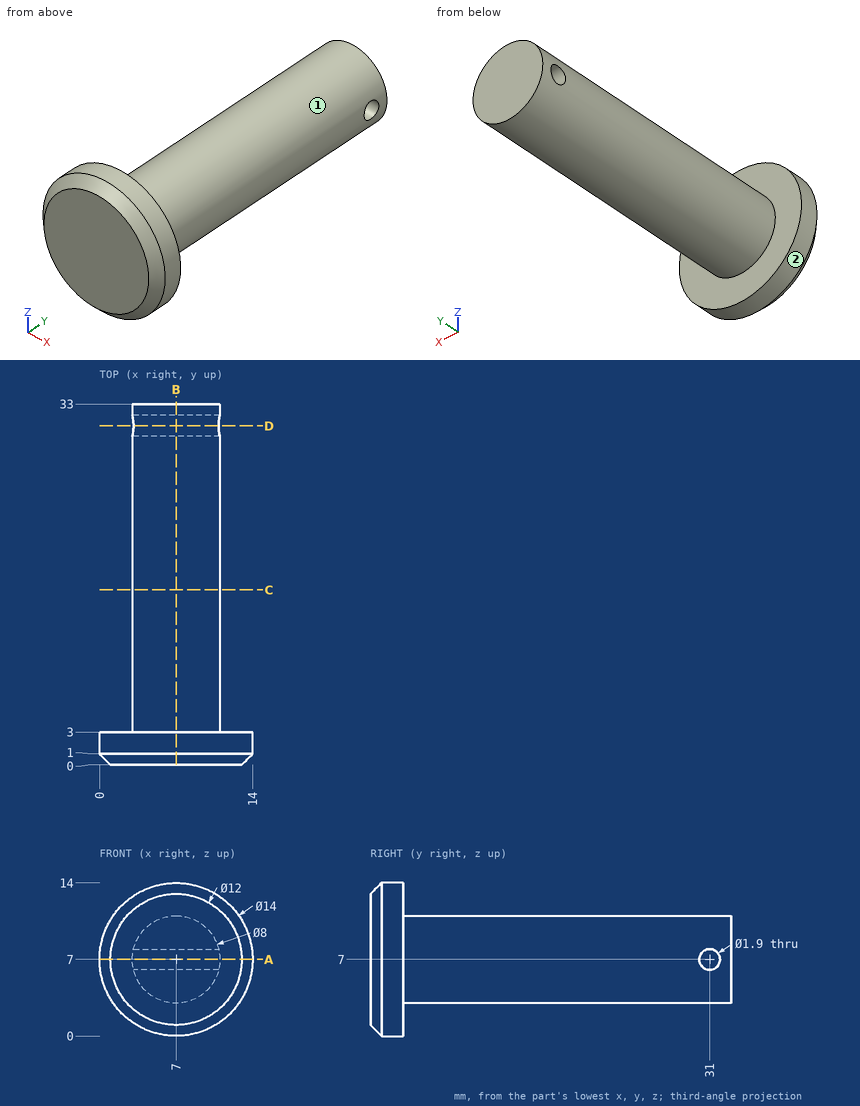
Study the drawing (mm; zero at the part's minimum x, y, z) and answer. A direction names the side the tool comes from. Coordinates: 2 decimals unless noted, no trailing zeros. Loops run counter-clockwise (first coordinate to the right, second up) from the corner with the lowest first, then second, coordinate; pieces in that order, holes last. Notation, with made-up numbers: (14, 21.25) -> (25, 21.25) arc R29 ccw to (25, 56.25) -> close; hole circle Ø9 at (27, 69). An arc over 180 degrees is marked (long way). Answer in a Markdown table with one row per item. Add a question column.
1. The part is cut by section A-A, the plane z = 7. Write down the section's boundary in (x, y).
2. The part is cut by section C-C, the plane y = 16. Write down the section's boundary in (x, z), then the cut area to 3 significant figures.
3. The part is cut by section B-B, the plane x = 7. Write down the section's boundary in (y, z).
4. The part is cut by section D-D, the plane y = 31. Write down the section's boundary in (x, z).
5. For the marked faces 1 and 2, determine the directions among +Z, -Z, +X, -X, +Y, -Y from which every point of the face is accessible in a straight line to the end or side of a thin tool.
6. Consider line 1 (Y direction, x = 6, z = 7); line 2 (Z direction, x = 6.75, y = 31); line 3 (Y direction, x = 12.5, z = 6.5). Determine where each line is inside the solid, lowest interval first. Write a range as [from, to].
7. Flat-ended cylindrical pins translate along their axes: P1, Ø2.5, axis at y = 31, z = 7, coming from the +X side; P2, Ø8, axis at x = 7.5, y = 14, coming from the +Z side; P3, Ø1.5, axis at x = 5, y = 17.5, coming from the +Z side. Find the tip coordinate at first contact, or state that the pin passes through.
Answer below:
| question | item | result |
|---|---|---|
| 1 | outline | (0, 1) -> (1, 0) -> (13, 0) -> (14, 1) -> (14, 3) -> (11, 3) -> (11, 30.05) -> (3, 30.05) -> (3, 3) -> (0, 3) -> close; (3, 31.95) -> (11, 31.95) -> (11, 33) -> (3, 33) -> close |
| 2 | outline | circle Ø8 at (7, 7) |
| 2 | area | 50.3 mm2 |
| 3 | outline | (0, 1) -> (1, 0) -> (3, 0) -> (3, 3) -> (33, 3) -> (33, 11) -> (3, 11) -> (3, 14) -> (1, 14) -> (0, 13) -> close; hole circle Ø1.9 at (31, 7) |
| 4 | outline | (3.11, 6.05) arc R4 ccw to (10.89, 6.05) -> close; (3.11, 7.95) -> (10.89, 7.95) arc R4 ccw to start |
| 5 | face 1 | +Y |
| 5 | face 2 | +Y, -Y |
| 6 | line 1 | [0, 30.05], [31.95, 33] |
| 6 | line 2 | [3.01, 6.05], [7.95, 10.99] |
| 6 | line 3 | [0, 3] |
| 7 | P1 | x = 11 |
| 7 | P2 | z = 11 |
| 7 | P3 | z = 10.8 |
